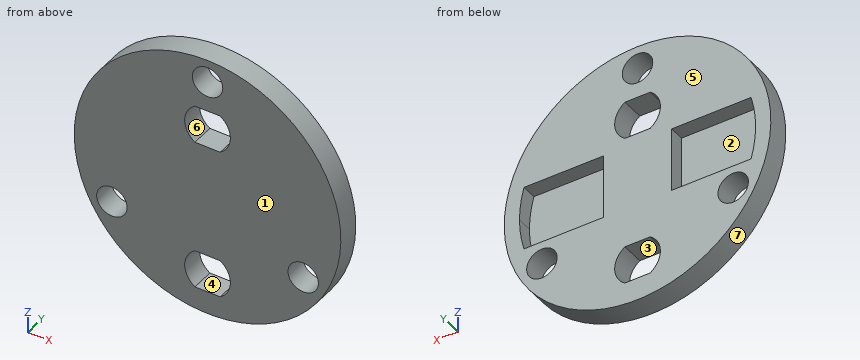
```python
from build123d import *

# Parameters (mm, degrees)
CROQUIS1_R              = 17.5
CROQUIS1_R_2            = 13.5
SALIENTE_EXTRUIR1_DEPTH = 3
CORTAR_EXTRUIR1_DEPTH   = 2
CROQUIS3_R              = 2
CORTAR_EXTRUIR2_DEPTH   = 25.929901725
CORTAR_EXTRUIR3_DEPTH   = 10


with BuildPart() as part:
    # Croquis1 → Saliente-Extruir1 (new body)
    with BuildSketch(Plane(origin=(0, 0, 0), x_dir=(1, 0, 0), z_dir=(0, 1, 0))):
        with Locations(Location((0, 0, 0), (0, 0, 270))):
            Circle(CROQUIS1_R)
        Circle(CROQUIS1_R_2, mode=Mode.SUBTRACT)
        Circle(CROQUIS1_R_2)
    extrude(amount=SALIENTE_EXTRUIR1_DEPTH)

    # Croquis2 → Cortar-Extruir1 (cut)
    with BuildSketch(Plane(origin=(0, 3, 0), x_dir=(1, 0, 0), z_dir=(0, 1, 0))):
        with BuildLine():
            Line((-15.5, 0), (-4.476086121, 0))
            Line((-4.476086121, 0), (-4.476086121, 4.25))
            Line((-4.476086121, 4.25), (-14.905955186, 4.25))
            ThreePointArc((-14.905955186, 4.25), (-15.350770427, 2.14565778), (-15.5, 0))
        make_face()
        with BuildLine():
            Line((-4.476086121, -4.25), (-4.476086121, 0))
            Line((-4.476086121, 0), (-15.5, 0))
            ThreePointArc((-15.5, 0), (-15.350770427, -2.14565778), (-14.905955186, -4.25))
            Line((-14.905955186, -4.25), (-4.476086121, -4.25))
        make_face()
        with BuildLine():
            ThreePointArc((15.5, 0), (15.350770427, 2.14565778), (14.905955186, 4.25))
            Line((14.905955186, 4.25), (4.476086121, 4.25))
            Line((4.476086121, 4.25), (4.476086121, -4.25))
            Line((4.476086121, -4.25), (14.905955186, -4.25))
            ThreePointArc((14.905955186, -4.25), (15.350770427, -2.14565778), (15.5, 0))
        make_face()
    extrude(amount=-CORTAR_EXTRUIR1_DEPTH, mode=Mode.SUBTRACT)

    # Croquis3 → Cortar-Extruir2 (cut, through all)
    with BuildSketch(Plane(origin=(0, 0, 0), x_dir=(-1, 0, 0), z_dir=(0, -1, 0))):
        with Locations(Location((0, -14.5, 0), (0, 0, 90))):
            Circle(CROQUIS3_R)
        with Locations(Location((12.557368355, 7.25, 0), (0, 0, 90))):
            Circle(CROQUIS3_R)
        with Locations(Location((-12.557368355, 7.25, 0), (0, 0, 90))):
            Circle(CROQUIS3_R)
    extrude(amount=-CORTAR_EXTRUIR2_DEPTH, mode=Mode.SUBTRACT)

    # Croquis4 → Cortar-Extruir3 (cut)
    with BuildSketch(Plane(origin=(0, 0, 0), x_dir=(-1, 0, 0), z_dir=(0, -1, 0))):
        with BuildLine():
            Line((1.658312395, 14.5), (-1.658312395, 14.5))
            ThreePointArc((-1.658312395, 14.5), (-3, 12), (-1.658312395, 9.5))
            Line((-1.658312395, 9.5), (1.658312395, 9.5))
            ThreePointArc((1.658312395, 9.5), (3, 12), (1.658312395, 14.5))
        make_face()
        with BuildLine():
            Line((1.658312395, -5.5), (-1.658312395, -5.5))
            ThreePointArc((-1.658312395, -5.5), (-3, -8), (-1.658312395, -10.5))
            Line((-1.658312395, -10.5), (1.658312395, -10.5))
            ThreePointArc((1.658312395, -10.5), (3, -8), (1.658312395, -5.5))
        make_face()
    extrude(amount=-CORTAR_EXTRUIR3_DEPTH, mode=Mode.SUBTRACT)


solid = part.part
```
Geometry: final body of the model. Coordinates: model frame, mm. Face numbers are marked on the shaded views. A direction names the side the tool comes from. Round coordinates to 2 decimals unless told otherwise and drop trailing zeros. Loops run counter-clockwise (first coordinate to the right, second up) from the corner with the lowest first, then second, coordinate; pieces in that order, holes last.
Item 1: Line query: L1, parallel to Z at x = -2.5, y = 1.5; L2, parallel to X at y = 2.4, z = -7.25; L3, parallel to Z at x = -1, y = 1.25. Output: solid intervals per line, ascending.
Checked values:
L1: z = -17.32 to -13.66, -10.34 to 6.34, 9.66 to 17.32
L2: x = -15.93 to -14.56, -10.56 to 10.56, 14.56 to 15.93
L3: z = -17.47 to -14.5, -9.5 to 5.5, 10.5 to 12.77, 16.23 to 17.47
Item 2: Section A-A, the plane x = 0. Output: boundary loops of the cut face in (y, z), plus the area to 3 significant figures.
Checked values:
outline: (0, -17.5) - (3, -17.5) - (3, -14.5) - (0, -14.5) - close; (0, -9.5) - (3, -9.5) - (3, 5.5) - (0, 5.5) - close; (0, 10.5) - (3, 10.5) - (3, 12.5) - (0, 12.5) - close; (0, 16.5) - (3, 16.5) - (3, 17.5) - (0, 17.5) - close
area: 63.0 mm2
Item 3: Section C-C, the plane y = 1.85. Output: boundary loops of the cut face in (x, z).
Checked values:
outline: circle Ø35 at (0, 0); hole (-14.91, -4.25) - (-4.48, -4.25) - (-4.48, 4.25) - (-14.91, 4.25) arc R15.5 ccw to start; hole circle Ø4 at (-12.56, -7.25); hole circle Ø4 at (0, 14.5); hole (-1.66, -14.5) - (1.66, -14.5) arc R3 ccw to (1.66, -9.5) - (-1.66, -9.5) arc R3 ccw to start; hole (-1.66, 5.5) - (1.66, 5.5) arc R3 ccw to (1.66, 10.5) - (-1.66, 10.5) arc R3 ccw to start; hole (4.48, -4.25) - (14.91, -4.25) arc R15.5 ccw to (14.91, 4.25) - (4.48, 4.25) - close; hole circle Ø4 at (12.56, -7.25)
Item 4: Mould query, pull axis Z, two halves, no side actions, for the marked faces 4, 5, 6 and 7. Classes: released by +Z, released by -Z, zero draft, split by the parting line, or undercut.
Checked values:
face 4: undercut
face 5: zero draft
face 6: undercut
face 7: split by the parting line
Item 5: Section D-D, the plane z = -7.25. Output: boundary loops of the cut face in (x, y).
Checked values:
outline: (-15.93, 0) - (-14.56, 0) - (-14.56, 3) - (-15.93, 3) - close; (-10.56, 0) - (10.56, 0) - (10.56, 3) - (-10.56, 3) - close; (14.56, 0) - (15.93, 0) - (15.93, 3) - (14.56, 3) - close
Item 6: Contact query for flat-ended pins moving along their axis: P1, Ø0.6, axis at x = -9, y = 2.5, coming from the -Z side; P2, Ø0.6, axis at x = 7.5, y = 2.5, coming from the -Z side; P3, Ø4.5, axis at x = 8, z = 0.5, coming from the +Y side; P4, Ø2.5, axis at x = 0, z = 14.5, coming from the -Y side. Output: stop coordinate, or through.
Checked values:
P1: stops at z = -15.18
P2: stops at z = -15.95
P3: stops at y = 1
P4: passes through
Item 7: Reachability of the marked faces 1, 2 and 3 from +Z, -Z, +X, -X, +Y, -Y: full face, straight path, thin tool, end or side. Return the list, or none.
Checked values:
face 1: +Z, -Z, +X, -X, -Y
face 2: +Y
face 3: +Y, -Y
Item 8: Section B-B, the plane z = 8. Output: boundary loops of the cut face in (x, y), plus the area to 3 significant figures.
Checked values:
outline: (-15.56, 0) - (-3, 0) - (-3, 3) - (-15.56, 3) - close; (3, 0) - (15.56, 0) - (15.56, 3) - (3, 3) - close
area: 75.4 mm2
